Part model, mm, in its own coordinate system. A direction names the side the tool comes from. Round coordinates to 2 decimals unless told otherwise and drop trailing zeros. Loops run counter-clockwise (first coordinate to the right, second up) from the corner with the lowest first, then second, coordinate; pieces in that order, holes last. Notation, with made-up numbers: (-5.5, -15) - (36.5, -15) arc R19 cw to (36.5, 1) - close; hole circle Ø9 at (-20, 89). An arc over 180 degrees is marked (long way). Put each result on its own line as item: value.
from build123d import *

# Parameters (mm, degrees)
F0_R     = 44.746468
F1_DEPTH = 177.8
F2_T     = -2.54


with BuildPart() as f1:
    # F0 (on Top) → F1 (new body)
    with BuildSketch(Plane.XY):
        Circle(F0_R)
    extrude(amount=F1_DEPTH)

    # F2
    f2_openings = [f1.faces().sort_by_distance(p)[0] for p in [
        (0, 0, 177.8),
    ]]
    offset(amount=F2_T, openings=f2_openings)

    # F3: F1 across plane


with BuildPart() as f1_1:
    add(f1.part)
    add(f1.part.mirror(Plane.XY))


solid = f1_1.part
1. Tool access for faces 4 (the flat face through (-27, -33, -177.8)), 5 (the cylindrical face through (-9.15, -41.203, 88.943)), 6 (the flat face through (-1, 1, -2.54)): list every direction of +Z, -Z, +X, -X, +Y, -Y with a clear straight run to the whole face (end or side of a thin tool).
A:
face 4: -Z, +X, -X, +Y, -Y
face 5: +Z
face 6: -Z
2. Two-plate mould, pull along Y, no slides. Class faces 1 (the flat face through (-1, 1, 2.54)), 2 (the flat face through (-27, -33, 177.8)), 3 (the cylindrical face through (-35.509, -27.228, 2.489)): pulls with the +Y half, pulls with the -Y half, needs draft (parallel to the pull), parting line crosses it, or undercut.
A:
face 1: undercut
face 2: needs draft
face 3: parting line crosses it
3. Band-saw the part on C-C (z = -90.5). List the corners of the cut face in (x, y), plus the area to 3 significant figures.
A:
outline: circle Ø89.49 at (0, 0); hole circle Ø84.41 at (0, 0)
area: 694 mm²
4. Probe line 1 along Y through (x, z) = (0, -59); line 2 along Z through (x, y) = (1, 2); line 3 along X through (y, z) = (1, -121). List the from-to ranges inside material, lowest first. Write a range as [from, to].
A:
line 1: y = [-44.75, -42.21], [42.21, 44.75]
line 2: z = [-2.54, 2.54]
line 3: x = [-44.74, -42.19], [42.19, 44.74]
5. Band-saw the part on A-A (x = 0). List the corners of the cut face in (y, z).
A:
outline: (-44.75, -177.8) - (-42.21, -177.8) - (-42.21, -2.54) - (42.21, -2.54) - (42.21, -177.8) - (44.75, -177.8) - (44.75, 177.8) - (42.21, 177.8) - (42.21, 2.54) - (-42.21, 2.54) - (-42.21, 177.8) - (-44.75, 177.8) - close
6. Pin check, flat tips, straight feed: P1, Ø10, axis at x = -11, y = 6, coming from the +Z side; P2, Ø2, axis at y = 18.5, z = -64.5, coming from the -X side; P3, Ø1, axis at x = -29, y = 15, coming from the -Z side. Stop position of each tip, or through.
A:
P1: stops at z = 2.54
P2: stops at x = -41.18
P3: stops at z = -2.54
